from build123d import *

# Parameters (mm, degrees)
SKETCH1_R                           = 50
SKETCH1_R_2                         = 15
BOSS_EXTRUDE2_DEPTH                 = 60
SKETCH1_3_R                         = 15
BOSS_EXTRUDE3_DEPTH                 = 600
CUT_EXTRUDE1_REACH                  = 606.152
CUT_EXTRUDE1_END_RADIUS             = 15
SKETCH2_W                           = 35
SKETCH2_H                           = 7.5
CUT_EXTRUDE1_DIRECTION_2_REACH      = 606.152
CUT_EXTRUDE1_DIRECTION_2_END_RADIUS = 15
CUT_EXTRUDE2_REACH                  = 606.152
SKETCH3_R                           = 5
CUT_EXTRUDE2_DIRECTION_2_REACH      = 606.152


with BuildPart() as part:
    # Sketch1 → Boss-Extrude2 (new body)
    # profile 1 of 2: a face of its own
    with BuildSketch(Plane(origin=(0, 0, 0), x_dir=(0, 0, -1), z_dir=(1, 0, 0))):
        Circle(SKETCH1_R)
        Circle(SKETCH1_R_2, mode=Mode.SUBTRACT)
    # profile 2 of 2: a face of its own
    with BuildSketch(Plane(origin=(0, 0, 0), x_dir=(0, 0, -1), z_dir=(1, 0, 0))):
        Circle(SKETCH1_R_2)
    extrude(amount=BOSS_EXTRUDE2_DEPTH)

    # Sketch1<3> → Boss-Extrude3 (add)
    with BuildSketch(Plane(origin=(0, 0, 0), x_dir=(0, 0, -1), z_dir=(1, 0, 0))):
        Circle(SKETCH1_3_R)
    extrude(amount=BOSS_EXTRUDE3_DEPTH)

    # Cut-Extrude1: up to this cylinder (the profile starts inside it)
    cut_extrude1_end = Plane(origin=(582.5, 0, 0), z_dir=(-1, 0, 0)) * Cylinder(CUT_EXTRUDE1_END_RADIUS, 1243.304, mode=Mode.PRIVATE)
    # Sketch2 → Cut-Extrude1 (cut, up to the surface)
    with BuildSketch(Plane(origin=(0, 0, 0), x_dir=(1, 0, 0), z_dir=(0, 1, 0)), mode=Mode.PRIVATE) as cut_extrude1_sk1:
        with Locations((582.5, 11.25)):
            Rectangle(SKETCH2_W, SKETCH2_H)
    cut_extrude1_tool1 = extrude(cut_extrude1_sk1.sketch, amount=-CUT_EXTRUDE1_REACH, mode=Mode.PRIVATE) & cut_extrude1_end
    add(cut_extrude1_tool1.solids().sort_by_distance((582.5, 0, -11.25))[0], mode=Mode.SUBTRACT)
    # Sketch2 → Cut-Extrude1 (cut, up to the surface)
    with BuildSketch(Plane(origin=(0, 0, 0), x_dir=(1, 0, 0), z_dir=(0, 1, 0)), mode=Mode.PRIVATE) as cut_extrude1_sk2:
        with Locations((582.5, -11.25)):
            Rectangle(SKETCH2_W, SKETCH2_H)
    cut_extrude1_tool2 = extrude(cut_extrude1_sk2.sketch, amount=-CUT_EXTRUDE1_REACH, mode=Mode.PRIVATE) & cut_extrude1_end
    add(cut_extrude1_tool2.solids().sort_by_distance((582.5, 0, 11.25))[0], mode=Mode.SUBTRACT)

    # Cut-Extrude1 direction 2: up to this cylinder (the profile starts inside it)
    cut_extrude1_direction_2_end = Plane(origin=(582.5, 0, 0), z_dir=(-1, 0, 0)) * Cylinder(CUT_EXTRUDE1_DIRECTION_2_END_RADIUS, 1243.304, mode=Mode.PRIVATE)
    # Sketch2 → Cut-Extrude1 direction 2 (cut, up to the surface)
    with BuildSketch(Plane(origin=(0, 0, 0), x_dir=(1, 0, 0), z_dir=(0, 1, 0)), mode=Mode.PRIVATE) as cut_extrude1_direction_2_sk1:
        with Locations((582.5, 11.25)):
            Rectangle(SKETCH2_W, SKETCH2_H)
    cut_extrude1_direction_2_tool1 = extrude(cut_extrude1_direction_2_sk1.sketch, amount=CUT_EXTRUDE1_DIRECTION_2_REACH, mode=Mode.PRIVATE) & cut_extrude1_direction_2_end
    add(cut_extrude1_direction_2_tool1.solids().sort_by_distance((582.5, 0, -11.25))[0], mode=Mode.SUBTRACT)
    # Sketch2 → Cut-Extrude1 direction 2 (cut, up to the surface)
    with BuildSketch(Plane(origin=(0, 0, 0), x_dir=(1, 0, 0), z_dir=(0, 1, 0)), mode=Mode.PRIVATE) as cut_extrude1_direction_2_sk2:
        with Locations((582.5, -11.25)):
            Rectangle(SKETCH2_W, SKETCH2_H)
    cut_extrude1_direction_2_tool2 = extrude(cut_extrude1_direction_2_sk2.sketch, amount=CUT_EXTRUDE1_DIRECTION_2_REACH, mode=Mode.PRIVATE) & cut_extrude1_direction_2_end
    add(cut_extrude1_direction_2_tool2.solids().sort_by_distance((582.5, 0, 11.25))[0], mode=Mode.SUBTRACT)

    # Sketch3 → Cut-Extrude2 (cut, up to next)
    with BuildSketch(Plane.XY, mode=Mode.PRIVATE) as cut_extrude2_sk1:
        with Locations(Location((585, 0, 0), (0, 0, 180))):
            Circle(SKETCH3_R)
    cut_extrude2_tool1 = extrude(cut_extrude2_sk1.sketch, amount=-CUT_EXTRUDE2_REACH, mode=Mode.PRIVATE) & part.part
    add(cut_extrude2_tool1.solids().sort_by_distance((585, 0, 0))[0], mode=Mode.SUBTRACT)

    # Sketch3 → Cut-Extrude2 direction 2 (cut, up to next)
    with BuildSketch(Plane.XY, mode=Mode.PRIVATE) as cut_extrude2_direction_2_sk1:
        with Locations(Location((585, 0, 0), (0, 0, 180))):
            Circle(SKETCH3_R)
    cut_extrude2_direction_2_tool1 = extrude(cut_extrude2_direction_2_sk1.sketch, amount=CUT_EXTRUDE2_DIRECTION_2_REACH, mode=Mode.PRIVATE) & part.part
    add(cut_extrude2_direction_2_tool1.solids().sort_by_distance((585, 0, 0))[0], mode=Mode.SUBTRACT)


solid = part.part
Check sheet for the modelled part. Datum: model origin and axes. Units: mm. A direction names the side the tool comes from. Give positions to 0.01 mm unless a question says otherwise; leave off trailing zeros. Loops run counter-clockwise (first coordinate to the right, second up) from the corner with the lowest first, then second, coordinate; pieces in that order, holes last. Notation, with made-up numbers: M 3,-2.75 L 36,-2.75 A17 ccw 36,10.25 Z; hole C -16,77.25 d11. An arc over 180 degrees is marked long. Answer as a JSON object with one key per item and string values. Group by question number.
Q1. Cross-section at D-D on x = 289. Record the cut outline in (y, z).
Q2. Material ranges on line 1 along X through (y, z) = (14, 32); line 2 along Y through (x, z) = (585, 0.25); line 3 along Y through (x, z) = (585, -2), recorded low to high. Write a range as [from, to].
Q3. Cross-section at A-A on x = 585. Record the cut outline in (y, z), then the cut area to 3 significant figures.
Q4. Cross-section at B-B on z = 0. Record the cut outline in (x, y), then the cut area to 3 significant figures.
Q5. Go/stop test with flat-tipped pins: P1, Ø6, axis at y = 31.5, z = 20.5, coming from the +X side; P2, Ø16, axis at x = 585, y = 0, coming from the -Z side; P3, Ø6, axis at y = -6, z = 13, coming from the +X side. Record where each tip stops, or that it passes through.
Q6. Cross-section at C-C on y = 0. Record the cut outline in (x, z), then the cut area to 3 significant figures.
Q7. Release check for a two-part mould opening along X. For faces 1 (the flat face through (578, 0, 7.5)), 2 (the cylindrical face through (580.381, 1.915, 0.105)), 3 (the flat face through (0, 1, 1)) record: released by +X, released by -X, zero draft, split by the parting line, or undercut.
Q8. Access from +Z, -Z, +X, -X, +Y, -Y to the whole of each face (thin tool, end or side, straight path). Record for faces 4 (the cylindrical face through (29.58, 15.02, -47.69)), 5 (the flat face through (578, 0, -7.5)), 6 (the flat face through (60, -10, 12)).
Evaluation:
{
 "1": {"outline": "C 0,0 d30"},
 "2": {"line 1": "x = [0, 60]", "line 2": "y = [-15, -5], [5, 15]", "line 3": "y = [-14.87, -5], [5, 14.87]"},
 "3": {"outline": "M -12.99,-7.5 L -5,-7.5 L -5,7.5 L -12.99,7.5 A15 ccw Z; M 5,-7.5 L 12.99,-7.5 A15 ccw 12.99,7.5 L 5,7.5 Z", "area": "280 mm2"},
 "4": {"outline": "M 0,-50 L 60,-50 L 60,-15 L 600,-15 L 600,15 L 60,15 L 60,50 L 0,50 Z; hole C 585,0 d10", "area": "22,100 mm2"},
 "5": {"P1": "stops at x = 60", "P2": "stops at z = -7.5", "P3": "stops at x = 565"},
 "6": {"outline": "M 0,-50 L 60,-50 L 60,-15 L 565,-15 L 565,-7.5 L 580,-7.5 L 580,7.5 L 565,7.5 L 565,15 L 60,15 L 60,50 L 0,50 Z; M 590,-7.5 L 600,-7.5 L 600,7.5 L 590,7.5 Z", "area": "21,500 mm2"},
 "7": {"face 1": "zero draft", "face 2": "undercut", "face 3": "released by -X"},
 "8": {"face 4": "+X, -X", "face 5": "-Z, +X, +Y, -Y", "face 6": "+X"}
}
